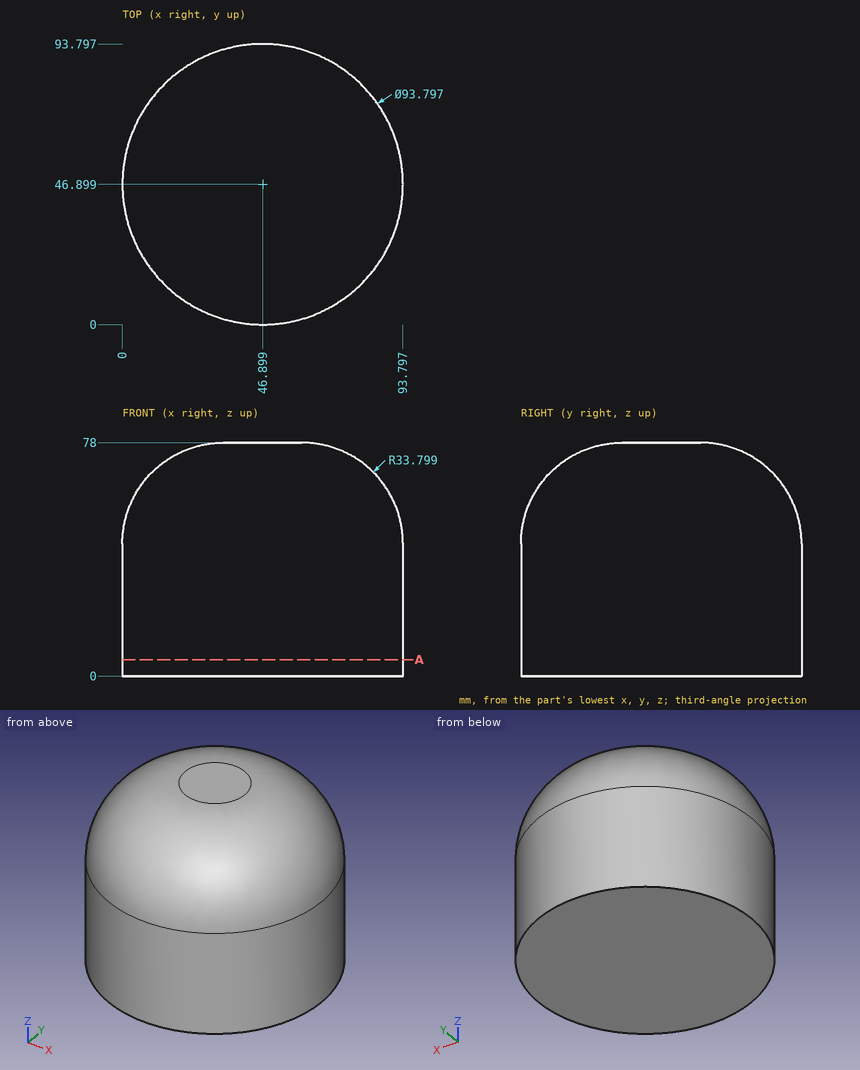
Geometry: see drawing. Coordinates: mm, zero at the bounding-box minimum. Give positions to 0.01 mm unless a question says otherwise; leave off trailing zeros. Loops run counter-clockwise (first coordinate to the right, second up) from the corner with the lowest first, then second, coordinate; pieces in that order, holes last. Notation, with made-up numbers: (-18.75, 23) - (-8.75, 23) arc R19 cw to (-8.75, 54) - close; hole circle Ø1 at (43.5, 74.5). An arc over 180 degrees is marked (long way). Use CSV: the item, a comma, the result in double quotes. Start each with the question number.
1. Pin query (flat end, axial travel): pin 1 (10 mm diameter, centred on x = 42, z = 66.5, fed in from +Y); pin 2 (8 mm diameter, centred on x = 66, z = 16.5, fed in from +Y); pin 3 (1.5 mm diameter, centred on y = 41, z = 56.5, fed in from +X); pin 4 (4 mm diameter, centred on x = 21.5, y = 42.5, fed in from -Z). Return the tip coordinate at first contact, or that it passes through.
2. Ray query, L1, parallel to Y at x = 49, z = 47.5; L2, parallel to Y at x = 68.5, z = 37.5 (1 decimal); L3, parallel to X at y = 11, z = 58 (1 decimal). Return the intervals inside material, ascending.
3. Section A-A (z = 5.5). Output: boundary loops of the cut face in (x, y).
Response:
1,pin 1,"y = 88.8"
1,pin 2,"y = 91.3"
1,pin 3,"x = 91.39"
1,pin 4,"z = 0"
2,L1,"0.21 to 93.59"
2,L2,"5.3 to 88.5"
2,L3,"21.5 to 72.3"
3,outline,"circle Ø93.8 at (46.9, 46.9)"
